```python
from build123d import *

# Parameters (mm, degrees)
CHAMFER_1_SIZE         = 1
HOLE_WIZARD_M4_1_D     = 3.3
HOLE_WIZARD_M4_1_DEPTH = 10
HOLE_WIZARD_M4_1_TIP   = 0.991420021


with BuildPart() as part:
    # 草图1 → 旋转1 (revolve)
    with BuildSketch(Plane.XY, mode=Mode.PRIVATE) as revolve_1_sk:
        Polygon((0, 0), (-6, 0), (-6, 15), (-4, 15), (-4, 20), (-10, 20), (-10, 25), (0, 25), align=None)
    revolve(revolve_1_sk.sketch.rotate(Axis((0, -198.13008407, 0), (0, 1, 0)), 180), axis=Axis((0, -198.13008407, 0), (0, 1, 0)))

    # 倒角1
    chamfer_1_edges = [part.edges().sort_by_distance(p)[0] for p in [
        (-6, 0, 0),
    ]]
    chamfer(chamfer_1_edges, length=CHAMFER_1_SIZE)

    # M4 螺纹孔1
    with Locations(Plane(origin=(0, 25, 0), x_dir=(1, 0, 0), z_dir=(0, 1, 0))):
        with Locations((0, 0)):
            Hole(HOLE_WIZARD_M4_1_D / 2, depth=HOLE_WIZARD_M4_1_DEPTH)
            with Locations((0, 0, -(HOLE_WIZARD_M4_1_DEPTH + HOLE_WIZARD_M4_1_TIP / 2))):  # 118° drill point
                Cone(0, HOLE_WIZARD_M4_1_D / 2, HOLE_WIZARD_M4_1_TIP, mode=Mode.SUBTRACT)


solid = part.part
```
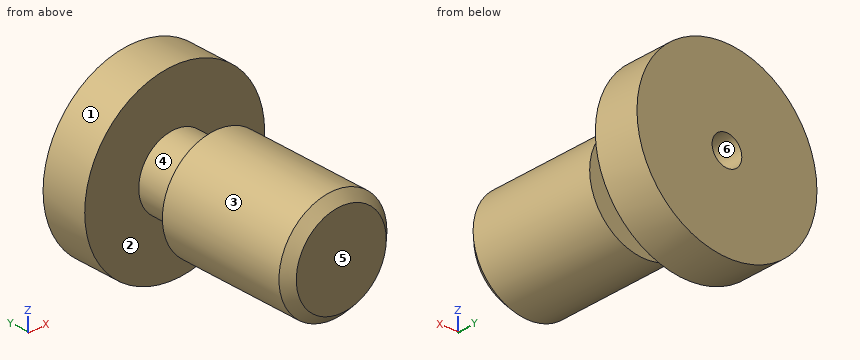
Here's how the part is built. I have some questions about the finished solid (model axes, mm). Face numbers are marked on the shaded views. A direction names the side the tool comes from. Coordinates: 2 decimals unless noted, no trailing zeros. Loops run counter-clockwise (first coordinate to the right, second up) from the corner with the lowest first, then second, coordinate; pieces in that order, holes last. Notation, with made-up numbers: M 19.25,84 L 54.25,84 A23 cw 54.25,112 Z; hole C -12.75,-33.75 d4. An arc over 180 degrees is marked long. One line per item, written item: value.
1. Will these pins go through, and if not, where does the flat tip stop? pin 1 Ø5 at (x, z) = (1.5, -6.5) entering from -Y; pin 2 Ø3 at (x, y) = (2.5, 22.5) entering from -Z; pin 3 Ø8 at (y, z) = (7, 3.5) entering from +X.
Geometry says:
pin 1: stops at y = 0
pin 2: stops at z = -9.95
pin 3: stops at x = 6
2. Imagine slicing it at D-D (x = 7.5). List the corners of the cut face in (y, z) for me, and give its area (3 significant figures).
Geometry says:
outline: M 20,-6.61 L 25,-6.61 L 25,6.61 L 20,6.61 Z
area: 66.1 mm2
3. On a 3-axis mill with a long thin cutter (end or side, diameter ignored), from which of +Z, -Z, +X, -X, +Y, -Y can I reach the whole of each face in a straight line? I mean the marked faces 1, 2 and 3. Say none if no direction works.
Geometry says:
face 1: +Y, -Y
face 2: none
face 3: -Y
4. Thinking about a two-plate mould opening in Z: for the marked faces 4, 5 and 6, which applies, +Z half, -Z half, draft (parallel to the pull), parting line (faces both ways), or undercut?
Geometry says:
face 4: parting line
face 5: draft
face 6: undercut
5. Imagine slicing it at A-A (y = 23). List the corners of the cut face in (x, z) for me.
Geometry says:
outline: C 0,0 d20; hole C 0,0 d3.3
6. Please list where these lines run through material, in increasing order: probe 1 along Z at (x, y) = (0, 19.75); probe 2 along Z at (x, y) = (0, 21); probe 3 along Y at (x, z) = (4.25, 2.5).
Geometry says:
probe 1: z = -4 to -1.65, 1.65 to 4
probe 2: z = -10 to -1.65, 1.65 to 10
probe 3: y = 0 to 15, 20 to 25
7. Imagine slicing it at B-B (y = 10.75). List the corners of the cut face in (x, z) for me.
Geometry says:
outline: C 0,0 d12
8. Imagine slicing it at C-C (z = -8). List the corners of the cut face in (x, y) for me.
Geometry says:
outline: M -6,20 L 6,20 L 6,25 L -6,25 Z
